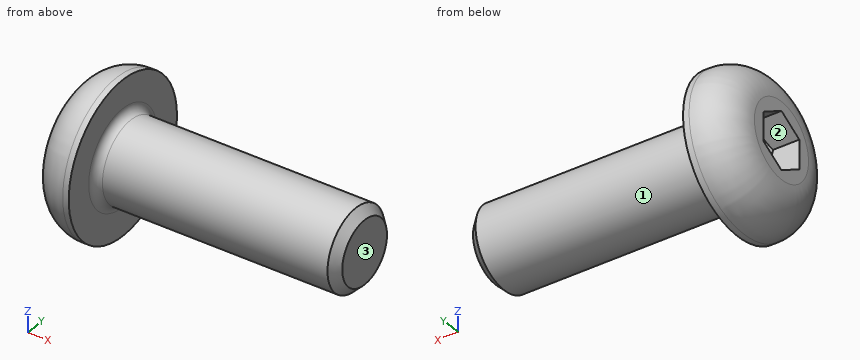
Autodesk Inventor part; units mm, degrees
ref_plane "Work Plane1" through (29, 0, 0) normal (0, -1, 0) x (1, 0, 0)
ref_plane "YZ Plane" through (0, 0, 0) normal (1, 0, 0) x (0, 1, 0)
ref_plane "XZ Plane" through (0, 0, 0) normal (0, 1, 0) x (-1, 0, 0)
sketch "Sketch1" plane through (0, 0, 0) normal (0, 0, 1) x (1, 0, 0)
  line L0 (-0.0667, 0) -> (12, 0)
  line L1 (12, 0) -> (12, 2)
  line L2 (12, 2) -> (2.1, 2)
  line L3 (2.1, 2) -> (1.6705, 2)
  line L4 (1.6705, 2) -> (0, 2)
  line L5 (0, 2) -> (0, 3.8)
  line L6 (0, 3.8) -> (-2.2, 3.8)
  line L7 (-2.2, 3.8) -> (-2.2, 1.4434)
  line L8 (-2.2, 1.4434) -> (-0.9, 1.4434)
  line L9 (-0.9, 1.4434) -> (-0.0667, 0)
  line L10 (-21, 0) -> (56, 0)
  line L11 (0, -1.6) -> (0, 9.6)
  line L12 (2.1, 2) -> (0, 2) construction
  dimension "d1" = 9.9
  dimension "d2" = 0.4295
  dimension "d3" = 2.2
  dimension "d4" = 1.3
  dimension "d5" = 60
  dimension "d6" = 4
  dimension "d7" = 4
  dimension "d8" = 2.8868
  dimension "d9" = 7.6
  dimension "d26" = 12
revolve "Body" add sketch "Sketch1" angle 360 about axis through (-0.0667, 0, 0) along (1, 0, 0)
sketch "Sketch2" plane through (-2.2, 0, 0) normal (-1, 0, 0) x (0, 0, 1)
  circle A0 centre (0, 0) radius 1.4434
  line L0 (0, -6.4663) -> (0, 6.4663)
  line L1 (-6.4663, 0) -> (6.4663, 0)
  line L2 (1.4434, 0) -> (0.7217, -1.25)
  line L3 (0.7217, -1.25) -> (-0.7217, -1.25)
  line L4 (-0.7217, -1.25) -> (-1.4434, 0)
  line L5 (-1.4434, 0) -> (-0.7217, 1.25)
  line L6 (-0.7217, 1.25) -> (0.7217, 1.25)
  line L7 (0.7217, 1.25) -> (1.4434, 0)
extrude "Slot" add sketch "Sketch2" against normal up to next contours L7 A0 | A0 L2 | L6 L0 A0 | A0 L0 L3 | L0 L6 A0 | A0 L3 L0 | L4 A0 | A0 L5
fillet "Fillet1" radius 1.9 1 edges at (-2.2, -3.8, 0)
thread "Thread"
chamfer "Chamfer1" distance 0.4294 distance2 0.4294 1 edges at (12, -2, 0) measured on face at (12, -1.1003, -0.6618)
ref_plane "Work Plane1" through (29, 0, 0) normal (0, -1, 0) x (1, 0, 0)
fillet "Fillet2" radius 0.4 1 edges at (0, -2, 0)
equation "\"d1\" = GEL"
equation "\"d3\" = KOH"
equation "\"d4\" = INTI"
equation "\"d6\" = GD"
equation "\"d7\" = BDM"
equation "\"d8\" = 1.1547 * SW"
equation "\"d9\" = KOD"
equation "\"d26\" = NLG"
equation "\"d30\" = R"
equation "\"d17\" = RR"
equation "\"d13\" = GEL"
equation "\"d15\" = -0.5 * SPD + 0.5 * GD"
equation "\"d16\" = GUL"
equation "\"GD\" = NND"
equation "\"NLG\" = 12"
equation "\"GEL\" = 9.9"
equation "\"KOD\" = 7.6"
equation "\"KOH\" = 2.2"
equation "\"INTI\" = 1.3"
equation "\"GAL\" = 0.61345 * PTC"
equation "\"GUL\" = 0.61345 * PTC"
equation "\"BDM\" = NND"
equation "\"SW\" = 2.5"
equation "\"RR\" = 1.9"
equation "\"SPD\" = NND - 1.2269 * PTC"
equation "\"R\" = 0.4"
equation "\"TOA\" = 30deg"
equation "\"GD1\" = THREADDIA - 1.2269 * PTC"
equation "\"THREADDIA\" = 4"
equation "\"PTC\" = 0.7"
equation "\"NND\" = 4"
equation "\"KOH1\" = 0.3"
equation "\"E0\" = 2.873"
properties part number "ISO 7380-1 - M4 x 12" material "Stainless Steel"
Here's how the part is built. I have some questions about the finished solid (model axes, mm). Face numbers are marked on the shaded views. A direction names the side the tool comes from. Coordinates: 2 decimals unless noted, no trailing zeros. Order: outer loops, then holes, each group sorted by start corner. A loop starts at its lowest first (then second) coordinate and runs counter-clockwise, first axis right, second up. Notation, with made-up numbers: (22.5, 58.5) -> (26.5, 58.5) arc R20 cw to (26.5, 85.5) -> close; hole circle Ø2 at (47, 64). An arc over 180 degrees is marked (long way). Answer in a Markdown table with one row per item.
(1) I want a section at A-A on x = 5.25. List the corners of the cut face in (y, z) for me.
Answer key:
| item | result |
|---|---|
| outline | circle Ø4 at (0, 0) |
(2) Please list where these lines run through material, in increasing order: probe 1 along Z at (x, y) = (-0.25, 0); probe 2 along X at (y, z) = (1, 0.75); probe 3 along Y at (x, z) = (4.5, -0.5).
Answer key:
| item | result |
|---|---|
| probe 1 | -3.8 to -0.32, 0.32 to 3.8 |
| probe 2 | -0.79 to 12 |
| probe 3 | -1.94 to 1.94 |
(3) On a 3-axis mill with a long thin cutter (end or side, diameter ignored), from which of +Z, -Z, +X, -X, +Y, -Y can I reach the whole of each face in a straight line? I mean the marked faces 1, 2 and 3. Say none if no direction works.
Answer key:
| item | result |
|---|---|
| face 1 | +X |
| face 2 | -X |
| face 3 | +Z, -Z, +X, +Y, -Y |
(4) Will these pins go through, and if not, where does the flat tip stop? pin 1 Ø1.5 at (y, z) = (-2.5, 0.5) entering from +X; pin 2 Ø3 at (x, y) = (5.5, 2.5) entering from +Z; pin 3 Ø1.6 at (x, z) = (-1.5, 0.5) entering from -Y.
Answer key:
| item | result |
|---|---|
| pin 1 | x = 11.77 |
| pin 2 | z = 1.73 |
| pin 3 | y = -3.74 |
